Could you check a few things on this model? Use its own coordinates, in mm. Coordinates: 2 decimals unless noted, no trailing zeros. Loops run counter-clockwise (first coordinate to the right, second up) from the corner with the lowest first, then second, coordinate; pieces in that order, holes last.
1) Imagine slicing it at A-A on z = -40. Please give me the cut outline in (x, y) (3 decimals).
2) Will these pins go through, and if not, where does the flat tip stop? P1, Ø2.5, axis at x = 0, z = -2.86, coming from the -Y side; P2, Ø1.5, axis at y = 1.5, z = -35, coming from the -X side; P3, Ø1.6, axis at y = 1.5, z = -24.5, coming from the +X side.
3) Imagine slicing it at C-C on y = 2.2. Please give me the cut outline in (x, z) (1 decimal).
4) If I drill on line 1 along X through (y, z) = (1.5, -60.5); line 2 along X through (y, z) = (0.3, -15.5) (3 decimals); line 3 along Z through (x, y) = (7.5, 2.5) (3 decimals), over which ranges is the centre line in solid material (lowest first)?
5) Imagine slicing it at B-B on x = 7. Please give me the cut outline in (y, z) (3 decimals).
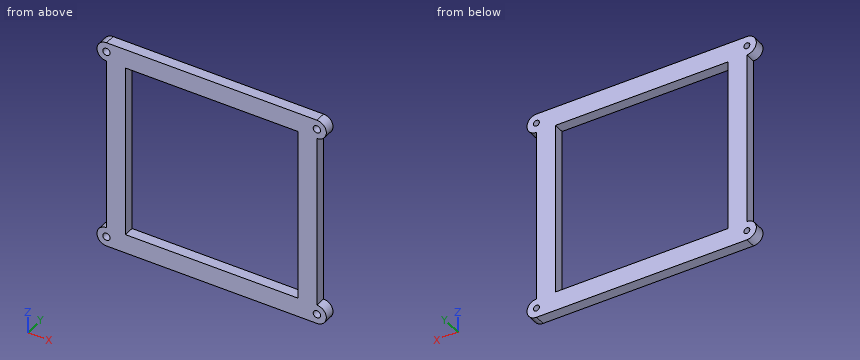
```python
from build123d import *

# Parameters (mm, degrees)
SKETCH1_W                = 52.07
SKETCH1_H                = 52.07
BOSS_EXTRUDE1_DEPTH      = 3.175
M2_CLEARANCE_HOLE1_D     = 2.2
M2_CLEARANCE_HOLE1_DEPTH = 3.048
M2_CLEARANCE_HOLE1_TIP   = 0.660946681


with BuildPart() as part:
    # Sketch1 → Boss-Extrude1 (new body)
    with BuildSketch(Plane(origin=(0, 0, 0), x_dir=(1, 0, 0), z_dir=(0, 1, 0))):
        with BuildLine():
            Line((0, 0), (63.5, 0))
            ThreePointArc((63.5, 0), (66.3575, 2.8575), (63.5, 5.715))
            Line((63.5, 5.715), (63.5, 57.785))
            ThreePointArc((63.5, 57.785), (66.3575, 60.6425), (63.5, 63.5))
            Line((63.5, 63.5), (0, 63.5))
            ThreePointArc((0, 63.5), (-2.8575, 60.6425), (0, 57.785))
            Line((0, 57.785), (0, 5.715))
            ThreePointArc((0, 5.715), (-2.8575, 2.8575), (0, 0))
        make_face()
        with Locations((31.75, 31.75)):
            Rectangle(SKETCH1_W, SKETCH1_H, mode=Mode.SUBTRACT)
    extrude(amount=BOSS_EXTRUDE1_DEPTH)

    # M2 Clearance Hole1
    with Locations(Plane(origin=(0, 0, 0), x_dir=(-1, 0, 0), z_dir=(0, -1, 0))):
        with Locations((-63.5, 60.6425), (0, 60.6425), (0, 2.8575), (-63.5, 2.8575)):
            Hole(M2_CLEARANCE_HOLE1_D / 2, depth=M2_CLEARANCE_HOLE1_DEPTH)
            with Locations((0, 0, -(M2_CLEARANCE_HOLE1_DEPTH + M2_CLEARANCE_HOLE1_TIP / 2))):  # 118° drill point
                Cone(0, M2_CLEARANCE_HOLE1_D / 2, M2_CLEARANCE_HOLE1_TIP, mode=Mode.SUBTRACT)


solid = part.part
```
Filled in:
1. outline: (0, 0) - (5.715, 0) - (5.715, 3.175) - (0, 3.175) - close; (57.785, 0) - (63.5, 0) - (63.5, 3.175) - (57.785, 3.175) - close
2. P1: stops at y = 0
2. P2: stops at x = 0
2. P3: stops at x = 63.5
3. outline: (0, -63.5) - (63.5, -63.5) arc R2.9 ccw to (63.5, -57.8) - (63.5, -5.7) arc R2.9 ccw to (63.5, 0) - (0, 0) arc R2.9 ccw to (0, -5.7) - (0, -57.8) arc R2.9 ccw to start; hole circle Ø2.2 at (0, -60.6); hole circle Ø2.2 at (0, -2.9); hole (5.7, -57.8) - (57.8, -57.8) - (57.8, -5.7) - (5.7, -5.7) - close; hole circle Ø2.2 at (63.5, -60.6); hole circle Ø2.2 at (63.5, -2.9)
4. line 1: x = -2.85 to -1.09, 1.09 to 62.41, 64.59 to 66.35
4. line 2: x = 0 to 5.715, 57.785 to 63.5
4. line 3: z = -63.5 to -57.785, -5.715 to 0
5. outline: (0, -63.5) - (3.175, -63.5) - (3.175, -57.785) - (0, -57.785) - close; (0, -5.715) - (3.175, -5.715) - (3.175, 0) - (0, 0) - close
